from build123d import *

# Parameters (mm, degrees)
F1_DEPTH  = 9.525
F3_DEPTH  = 63.5
F4_R      = 19.05
F5_DEPTH  = 9.526
F6_R      = 6.35
F7_DEPTH  = 31.75
F8_DEPTH  = 25.4
F9_R      = 6.35
F10_DEPTH = 25.4


with BuildPart() as f1:
    # F0 (on Front) → F1 (new body)
    with BuildSketch(Plane.XZ):
        with BuildLine():
            Line((-82.55, 12.7), (-82.55, -63.5))
            Line((-82.55, -63.5), (82.55, -63.5))
            Line((82.55, -63.5), (82.55, 0.801746))
            Line((82.55, 0.801746), (82.55, 12.7))
            Line((82.55, 12.7), (57.15, 12.7))
            ThreePointArc((57.15, 12.7), (39.189488, 20.139488), (31.75, 38.1))
            Line((31.75, 38.1), (31.75, 63.5))
            Line((31.75, 63.5), (-6.35, 63.5))
            Line((-6.35, 63.5), (-31.75, 63.5))
            Line((-31.75, 63.5), (-31.75, 38.1))
            ThreePointArc((-31.75, 38.1), (-39.189488, 20.139488), (-57.15, 12.7))
            Line((-57.15, 12.7), (-82.55, 12.7))
        make_face()
        with BuildLine():
            Line((-82.55, 20.29972), (-82.55, 12.7))
            Line((-82.55, 12.7), (-57.15, 12.7))
            ThreePointArc((-57.15, 12.7), (-39.189488, 20.139488), (-31.75, 38.1))
            Line((-31.75, 38.1), (-31.75, 63.5))
            Line((-31.75, 63.5), (-82.55, 63.5))
            Line((-82.55, 63.5), (-82.55, 20.29972))
        make_face()
        with BuildLine():
            Line((57.15, 12.7), (82.55, 12.7))
            Line((82.55, 12.7), (82.55, 63.5))
            Line((82.55, 63.5), (34.184467, 63.5))
            Line((34.184467, 63.5), (31.75, 63.5))
            Line((31.75, 63.5), (31.75, 38.1))
            ThreePointArc((31.75, 38.1), (39.189488, 20.139488), (57.15, 12.7))
        make_face()
    extrude(amount=F1_DEPTH)

    # F2 (on face) → F3 (join)
    with BuildSketch(Plane.XZ.offset(9.525)):
        with BuildLine():
            Line((-31.75, 63.5), (-82.55, 63.5))
            Line((-82.55, 63.5), (-82.55, 12.7))
            Line((-82.55, 12.7), (-57.15, 12.7))
            ThreePointArc((-57.15, 12.7), (-39.189488, 20.139488), (-31.75, 38.1))
            Line((-31.75, 38.1), (-31.75, 63.5))
        make_face()
        with BuildLine():
            Line((82.55, 12.7), (82.55, 63.5))
            Line((82.55, 63.5), (31.75, 63.5))
            Line((31.75, 63.5), (31.75, 38.1))
            ThreePointArc((31.75, 38.1), (39.189488, 20.139488), (57.15, 12.7))
            Line((57.15, 12.7), (82.55, 12.7))
        make_face()
    extrude(amount=F3_DEPTH)

    # F4 (on face) → F5 (cut, through all)
    with BuildSketch(Plane.XZ.offset(9.525)):
        Circle(F4_R)
    extrude(amount=-F5_DEPTH, mode=Mode.SUBTRACT)

    # F6 (on face) → F7 (cut)
    with BuildSketch(Plane.XZ.offset(73.025)):
        with Locations((-57.15, 38.1)):
            Circle(F6_R)
    extrude(amount=-F7_DEPTH, mode=Mode.SUBTRACT)

    # F6 (on face) → F8 (cut)
    with BuildSketch(Plane.XZ.offset(73.025)):
        with Locations((-57.15, 38.1)):
            Circle(F6_R)
    extrude(amount=-F8_DEPTH, mode=Mode.SUBTRACT)

    # F9 (on face) → F10 (cut)
    with BuildSketch(Plane.XZ.offset(73.025)):
        with Locations((57.15, 38.1)):
            Circle(F9_R)
    extrude(amount=-F10_DEPTH, mode=Mode.SUBTRACT)


solid = f1.part
Geometry: final body of the model. Coordinates: model frame, mm. A direction names the side the tool comes from. Coordinates: 2 decimals unless noted, no trailing zeros. Order: outer loops, then holes, each group sorted by start corner. A loop starts at its lowest first (then second) coordinate and runs counter-clockwise, first axis right, second up.
1) First-contact query: P1, Ø20.5, axis at x = -67, y = -50, coming from the -Z side; P2, Ø10, axis at x = 56.5, z = 37.5, coming from the -Y side (3 decimals); P3, Ø6.5, axis at x = -58, z = 39.5, coming from the -Y side (3 decimals); P4, Ø8, axis at x = 13.5, z = -5.5, coming from the -Y side. Flat tips, straight axial feed; report the tip coordinate or a pass-through.
Result sheet:
P1: stops at z = 12.7
P2: stops at y = -47.625
P3: stops at y = -41.275
P4: passes through
2) Section C-C (y = -28). Return loops of the section in (x, z), then the cut area to 3 significant figures.
Result sheet:
outline: (-82.55, 12.7) - (-57.15, 12.7) arc R25.4 ccw to (-31.75, 38.1) - (-31.75, 63.5) - (-82.55, 63.5) - close; (31.75, 38.1) arc R25.4 ccw to (57.15, 12.7) - (82.55, 12.7) - (82.55, 63.5) - (31.75, 63.5) - close
area: 4,880 mm2
3) Draft query along X for faces 1 (the flat face through (31.75, -41, 51)), 2 (the flat face through (-1, -5, -63.5)), 3 (the flat face through (-82.55, -36, 29)). Return one class per face: released by +X, released by -X, zero draft, split by the parting line, or undercut.
Result sheet:
face 1: undercut
face 2: zero draft
face 3: released by -X
4) Section D-D (z = 10). Return loops of the section in (x, y) (3 decimals), then the cut area to 3 significant figures.
Result sheet:
outline: (-82.55, -9.525) - (-16.214, -9.525) - (-16.214, 0) - (-82.55, 0) - close; (16.214, -9.525) - (82.55, -9.525) - (82.55, 0) - (16.214, 0) - close
area: 1,260 mm2
5) Section B-B (x = 0). Return loops of the section in (y, z) (3 decimals), then the cut area to 3 significant figures.
Result sheet:
outline: (-9.525, -63.5) - (0, -63.5) - (0, -19.05) - (-9.525, -19.05) - close; (-9.525, 19.05) - (0, 19.05) - (0, 63.5) - (-9.525, 63.5) - close
area: 847 mm2
6) Set-up query: faces 4 (the flat face through (-31.75, -41, 51)), 5 (the flat face through (-70, -41, 12.7)), 6 (the cylindrical face through (38.99, -40.83, 20.34)), 7 (the flat face through (-57, -41.275, 38)), 8 (the cylindrical face through (-15.12, -4.83, -11.59)). Return all of +Z, -Z, +X, -X, +Y, -Y with unobstructed straight access to the full face (end or side cutting, diameter ignored); none if empty.
Result sheet:
face 4: +Z, -Z, -Y
face 5: -Z, +X, -X, -Y
face 6: -Z, -Y
face 7: -Y
face 8: +Y, -Y
7) Ray query, probe 1 along Z at (x, y) = (57.15, -54.5); probe 2 along Y at (x, z) = (24, -25.5) (3 decimals); probe 3 along X at (y, z) = (-66.5, 22.5). Return the intervals inside material, ascending.
Result sheet:
probe 1: z = 12.7 to 31.75, 44.45 to 63.5
probe 2: y = -9.525 to 0
probe 3: x = -82.55 to -37.11, 37.11 to 82.55
8) Section A-A (y = -64). Return loops of the section in (x, z), then the cut area to 3 significant figures.
Result sheet:
outline: (-82.55, 12.7) - (-57.15, 12.7) arc R25.4 ccw to (-31.75, 38.1) - (-31.75, 63.5) - (-82.55, 63.5) - close; (31.75, 38.1) arc R25.4 ccw to (57.15, 12.7) - (82.55, 12.7) - (82.55, 63.5) - (31.75, 63.5) - close; hole circle Ø12.7 at (-57.15, 38.1); hole circle Ø12.7 at (57.15, 38.1)
area: 4,630 mm2
